Can you work these out from the model? Positions are in its coordinate system, mm. A direction names the side the tool comes from. Give positions to 0.01 mm unless a question says otherwise; leave off trailing zeros. Order: outer loops, then holes, each group sorted by start corner. A loop starts at its lowest first (then second) coordinate and runs counter-clockwise, first axis right, second up. Notation, with made-up numbers: M -23,33 L -1,33 A27 ccw -1,51 Z; hole C -3.5,75 d8. An arc over 180 degrees is marked long. Use a Markdown table: item, result. Add a question column.
from build123d import *

# Parameters (mm, degrees)
SKETCH1_W           = 106.8
SKETCH1_H           = 32.5
BOSS_EXTRUDE1_DEPTH = 4.79
SKETCH2_W           = 21.1
SKETCH2_H           = 26.3
BOSS_EXTRUDE2_DEPTH = 4.2
SKETCH3_W           = 15
SKETCH3_H           = 14.3
BOSS_EXTRUDE3_DEPTH = 9.2
SKETCH4_W           = 6.47
SKETCH4_H           = 11.45
BOSS_EXTRUDE4_DEPTH = 6
SKETCH5_R           = 1.375
CUT_EXTRUDE1_DEPTH  = 57.570862641
SKETCH6_W           = 7
SKETCH6_H           = 12.3
CUT_EXTRUDE2_DEPTH  = 12
SKETCH7_W           = 4.917083014
SKETCH7_H           = 8.943215518
CUT_EXTRUDE3_DEPTH  = 6


with BuildPart() as part:
    # Sketch1 → Boss-Extrude1 (new body)
    with BuildSketch(Plane.XY):
        Rectangle(SKETCH1_W, SKETCH1_H)
    extrude(amount=BOSS_EXTRUDE1_DEPTH)

    # Sketch2 → Boss-Extrude2 (add)
    with BuildSketch(Plane.XY.offset(4.79)):
        with Locations((-36.69, 0.014279692)):
            Rectangle(SKETCH2_W, SKETCH2_H)
    extrude(amount=BOSS_EXTRUDE2_DEPTH)

    # Sketch3 → Boss-Extrude3 (add)
    with BuildSketch(Plane.XY.offset(4.79)):
        with Locations((45.9, -0.1)):
            Rectangle(SKETCH3_W, SKETCH3_H)
    extrude(amount=BOSS_EXTRUDE3_DEPTH)

    # Sketch4 → Boss-Extrude4 (add)
    with BuildSketch(Plane.XY.offset(4.79)):
        with Locations((32.1, -8.63)):
            Rectangle(SKETCH4_W, SKETCH4_H)
    extrude(amount=BOSS_EXTRUDE4_DEPTH)

    # Sketch5 → Cut-Extrude1 (cut, through all)
    with BuildSketch(Plane.XY.offset(4.79)):
        with Locations((51.25, 13.12)):
            Circle(SKETCH5_R)
    extrude(amount=-CUT_EXTRUDE1_DEPTH, mode=Mode.SUBTRACT)

    # Sketch6 → Cut-Extrude2 (cut)
    with BuildSketch(Plane(origin=(53.4, 0, 0), x_dir=(0, 0, -1), z_dir=(1, 0, 0))):
        with Locations((-8.09, -0.1)):
            Rectangle(SKETCH6_W, SKETCH6_H)
    extrude(amount=-CUT_EXTRUDE2_DEPTH, mode=Mode.SUBTRACT)

    # Sketch7 → Cut-Extrude3 (cut)
    with BuildSketch(Plane(origin=(53.4, 0, 0), x_dir=(0, 0, -1), z_dir=(1, 0, 0))):
        with Locations((-2.131458493, 0)):
            Rectangle(SKETCH7_W, SKETCH7_H)
    extrude(amount=-CUT_EXTRUDE3_DEPTH, mode=Mode.SUBTRACT)


solid = part.part
1. If we section it at B-B, the plane z = 7: List the corners of the cut face in (x, y) for me (3 decimals), then the cut area to 3 significant figures.
2. If we section it at A-A, the plane x = 51.25: List the corners of the cut face in (y, z) for me (3 decimals).
3. If we section it at C-C, the plane z = 1.75: List the corners of the cut face in (x, y) for me (3 decimals), then the cut area to 3 significant figures.
4. We'd pull the mould along X, two halves only. Please class faces 6 (the face through (49.876, 13.18, 2.429)), 7 (the face through (-47.24, 0, 7)), 8 (the face through (-37, -13.136, 7)), 9 (the face through (53.4, -5, 4)): +X half, -X half, draft (parallel to the pull), parting line (faces both ways), or undercut.
5. I need wall thicknesses on L1, parallel to Y at x = 51.25, z = 1.65 (3 decimals); L2, parallel to X at y = 6, z = 8.75; L3, parallel to X at y = 4, z = 13. Which ranges of each line are inside material? Lowest first, please. Write a range as [from, to].
6. On a 3-axis mill with a long thin cutter (end or side, diameter ignored), from which of +Z, -Z, +X, -X, +Y, -Y can I reach the whole of each face in a straight line? I mean faces 1 (the face through (46, 7.05, 9)), 2 (the face through (45, 0, 4.59)), 3 (the face through (-37, 13.164, 7)), 4 (the face through (35.335, -9, 8)), 5 (the face through (50, 4.472, 2)). Say none if no direction works.
7. Will these pins go through, and if not, where does the flat tip stop? pin 1 (12 mm diameter, centred on x = 18.5, y = -7.5, fed in from -Z); pin 2 (2 mm diameter, centred on x = 45.5, z = 7.5, fed in from +Y); pin 3 (3 mm diameter, centred on x = -28.5, y = 6.5, fed in from +Z); pin 4 (2 mm diameter, centred on y = 6, z = 8, fed in from -X).
8. If we section it at D-D, the plane y = 8.5: List the corners of the cut face in (x, z) for me.
Geometry results:
| question | item | result |
|---|---|---|
| 1 | outline | M -47.24,-13.136 L -26.14,-13.136 L -26.14,13.164 L -47.24,13.164 Z; M 28.865,-14.355 L 35.335,-14.355 L 35.335,-2.905 L 28.865,-2.905 Z; M 38.4,-7.25 L 53.4,-7.25 L 53.4,-6.25 L 41.4,-6.25 L 41.4,6.05 L 53.4,6.05 L 53.4,7.05 L 38.4,7.05 Z |
| 1 | area | 696 mm^2 |
| 2 | outline | M -16.25,0 L -4.472,0 L -4.472,4.59 L -6.25,4.59 L -6.25,11.59 L 6.05,11.59 L 6.05,4.59 L 4.472,4.59 L 4.472,0 L 11.745,0 L 11.745,4.79 L 7.05,4.79 L 7.05,13.99 L -7.25,13.99 L -7.25,4.79 L -16.25,4.79 Z; M 14.495,0 L 16.25,0 L 16.25,4.79 L 14.495,4.79 Z |
| 3 | outline | M -53.4,-16.25 L 53.4,-16.25 L 53.4,-4.472 L 47.4,-4.472 L 47.4,4.472 L 53.4,4.472 L 53.4,16.25 L -53.4,16.25 Z; hole C 51.25,13.12 d2.75 |
| 3 | area | 3,410 mm^2 |
| 4 | face 6 | undercut |
| 4 | face 7 | -X half |
| 4 | face 8 | draft |
| 4 | face 9 | +X half |
| 5 | L1 | y = [-16.25, -4.472], [4.472, 11.745], [14.495, 16.25] |
| 5 | L2 | x = [-47.24, -26.14], [38.4, 41.4] |
| 5 | L3 | x = [38.4, 53.4] |
| 6 | face 1 | +Z, +X, +Y |
| 6 | face 2 | +X |
| 6 | face 3 | +Z, +X, -X, +Y |
| 6 | face 4 | +Z, +Y, -Y |
| 6 | face 5 | -Z, +X |
| 7 | pin 1 | stops at z = 0 |
| 7 | pin 2 | stops at y = 7.05 |
| 7 | pin 3 | stops at z = 8.99 |
| 7 | pin 4 | stops at x = -47.24 |
| 8 | outline | M -53.4,0 L 53.4,0 L 53.4,4.79 L -26.14,4.79 L -26.14,8.99 L -47.24,8.99 L -47.24,4.79 L -53.4,4.79 Z |
